CAD build for the part. Positions are in the model's coordinates, mm. Face numbers are marked on the shaded views. A direction names the side the tool comes from. Coordinates: 2 decimals unless noted, no trailing zeros. Loops run counter-clockwise (first coordinate to the right, second up) from the corner with the lowest first, then second, coordinate; pieces in that order, holes last. Notation, with made-up numbers: (-0.75, 3) -> (28.25, 3) arc R26 ccw to (28.25, 37) -> close; hole circle Ø7 at (8.25, 60.25). An arc over 180 degrees is marked (long way). Answer as CSV lines item,"result". Start each with the question number.
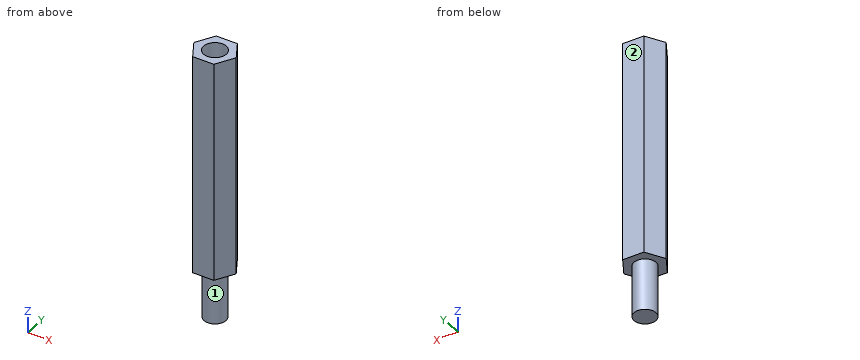
```python
from build123d import *

# Parameters (mm, degrees)
PAD_DEPTH    = 30
SKETCH001_R  = 1.55
POCKET_DEPTH = 15
SKETCH002_R  = 1.5
PAD001_DEPTH = 7


with BuildPart() as part:
    # Sketch → Pad (new body)
    with BuildSketch(Plane.XY):
        Polygon((2.886751, 0), (1.443376, 2.5), (-1.443376, 2.5), (-2.886751, 0), (-1.443376, -2.5), (1.443376, -2.5), align=None)
    extrude(amount=PAD_DEPTH)

    # Sketch001 (on Face8 of Pad) → Pocket (cut)
    with BuildSketch(Plane.XY.offset(30)):
        Circle(SKETCH001_R)
    extrude(amount=-POCKET_DEPTH, mode=Mode.SUBTRACT)

    # Sketch002 (on Face4 of Pocket) → Pad001 (join)
    with BuildSketch(Plane(origin=(0, 0, 0), x_dir=(1, 0, 0), z_dir=(0, 0, -1))):
        Circle(SKETCH002_R)
    extrude(amount=PAD001_DEPTH)


solid = part.part
```
Q1. Which spindle directions (+Z, -Z, +X, -X, +Y, -Y) get a long thin tool onto all of the face, cutting with end or side? Do the marked faces 1 and 2. Say none if no direction does.
Q2. Pin check, flat tips, straight feed: pin 1 Ø1 at (x, z) = (2, 2) entering from -Y; pin 2 Ø2.5 at (x, y) = (0, 0) entering from +Z. Stop position of each tip, or through.
Q3. Saw through at B-B (z = 8). List the corners of the cut face in (x, y).
Q4. Saw through at A-A (x = 0). List the corners of the cut face in (y, z), and give its area (4 significant figures).
Q5. Probe probe 1 along Y at (x, z) = (0.1, 27.5); probe 2 along Z at (x, y) = (0.45, -1.9); probe 3 along Z at (x, y) = (-0.4, 1.2). List the from-to ranges inside material, lowest first. Write a range as from..to.
Q6. Saw through at D-D (z = -4). List the corners of the cut face in (x, y), and give its area (3 significant figures).
Q7. Saw through at C-C (y = 0.4). List the corners of the cut face in (x, z), and give its area (3 significant figures).
Ans:
1,face 1,"-Z"
1,face 2,"+Z, -Z, +X, -X, +Y"
2,pin 1,"stops at y = -2.4"
2,pin 2,"stops at z = 15"
3,outline,"(-2.89, 0) -> (-1.44, -2.5) -> (1.44, -2.5) -> (2.89, 0) -> (1.44, 2.5) -> (-1.44, 2.5) -> close"
4,outline,"(-2.5, 0) -> (-1.5, 0) -> (-1.5, -7) -> (1.5, -7) -> (1.5, 0) -> (2.5, 0) -> (2.5, 30) -> (1.55, 30) -> (1.55, 15) -> (-1.55, 15) -> (-1.55, 30) -> (-2.5, 30) -> close"
4,area,"124.5 mm²"
5,probe 1,"y = -2.5..-1.55, 1.55..2.5"
5,probe 2,"z = 0..30"
5,probe 3,"z = -7..15"
6,outline,"circle Ø3 at (0, 0)"
6,area,"7.07 mm²"
7,outline,"(-2.66, 0) -> (-1.45, 0) -> (-1.45, -7) -> (1.45, -7) -> (1.45, 0) -> (2.66, 0) -> (2.66, 30) -> (1.5, 30) -> (1.5, 15) -> (-1.5, 15) -> (-1.5, 30) -> (-2.66, 30) -> close"
7,area,"135 mm²"
